The drawing under review shows one solid part. Ordinate dimensions are in mm from its lowest x, y, z. Round coordinates to 2 decimals unless told otherwise and drop trailing zeros. Order: outer loops, then holes, each group sorted by start corner. A loop starts at its lowest first (then second) coordinate and runs counter-clockwise, first axis right, second up. Notation, with made-up numbers: M -36,-28 L 3,-28 A20 ccw 3,-12 Z; hole C -37.75,76 d5. An arc over 180 degrees is marked long. Answer as a JSON object with one key per item and string values.
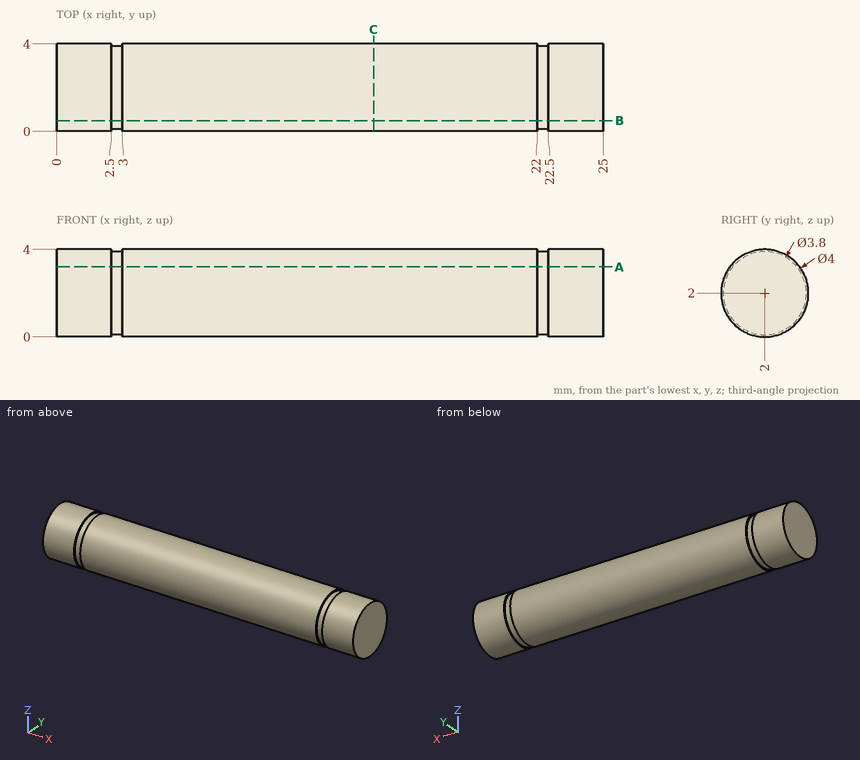
1) Add section C-C on x = 14.5. State the section outline as (y, z) points, and give its area (3 significant figures).
Geometry check:
{"outline": "C 2,2 d4", "area": "12.6 mm²"}
2) Add section A-A on z = 3.2. State the section outline as (x, y) points.
Geometry check:
{"outline": "M 0,0.4 L 2.5,0.4 L 2.5,0.53 L 3,0.53 L 3,0.4 L 22,0.4 L 22,0.53 L 22.5,0.53 L 22.5,0.4 L 25,0.4 L 25,3.6 L 22.5,3.6 L 22.5,3.47 L 22,3.47 L 22,3.6 L 3,3.6 L 3,3.47 L 2.5,3.47 L 2.5,3.6 L 0,3.6 Z"}
3) For L1, parallel to X at y = 0.2, z = 1.3; L2, parallel to Y at x = 20.25, z = 2.1; L3, parallel to Z at x = 20, y = 2.15, list the stretches that pass through material, from the lowest coordinate up.
Geometry check:
{"L1": "x = 0 to 2.5, 3 to 22, 22.5 to 25", "L2": "y = 0 to 4", "L3": "z = 0.01 to 3.99"}
4) Add section B-B on y = 0.5. State the section outline as (x, z) points.
Geometry check:
{"outline": "M 0,0.68 L 2.5,0.68 L 2.5,0.83 L 3,0.83 L 3,0.68 L 22,0.68 L 22,0.83 L 22.5,0.83 L 22.5,0.68 L 25,0.68 L 25,3.32 L 22.5,3.32 L 22.5,3.17 L 22,3.17 L 22,3.32 L 3,3.32 L 3,3.17 L 2.5,3.17 L 2.5,3.32 L 0,3.32 Z"}
